Work out the finished part from the listing and answer in its coordinate system (mm). A direction names the side the tool comes from. Give positions to 0.01 mm unless a question says otherwise; leave off trailing zeros. Loops run counter-clockwise (first coordinate to the right, second up) from the corner with the lowest first, then second, coordinate; pieces in that order, holes last. Notation, with made-up numbers: (22, 29.5) - (52, 29.5) arc R6 cw to (52, 33.5) - close; hole circle Ø9 at (48, -1). An arc over 180 degrees is marked (long way). One line per item, written item: value.
from build123d import *

# Parameters (mm, degrees)
SKETCH_R  = 1.8288
PAD_DEPTH = 3


with BuildPart() as part:
    # Sketch → Pad (new body)
    with BuildSketch(Plane.XY):
        with BuildLine():
            Line((0, 100.6), (0, 1))
            ThreePointArc((0, 1), (0.292893, 0.292893), (1, 0))
            Line((1, 0), (14.748, 0))
            ThreePointArc((14.748, 0), (15.455107, 0.292893), (15.748, 1))
            Line((15.748, 12.7), (15.748, 1))
            ThreePointArc((22.352, 12.7), (19.05, 16.002), (15.748, 12.7))
            Line((22.352, 12.7), (22.352, 1))
            ThreePointArc((22.352, 1), (22.644893, 0.292893), (23.352, 0))
            Line((23.352, 0), (74.748, 0))
            ThreePointArc((74.748, 0), (75.455107, 0.292893), (75.748, 1))
            Line((75.748, 12.7), (75.748, 1))
            ThreePointArc((82.352, 12.7), (79.05, 16.002), (75.748, 12.7))
            Line((82.352, 12.7), (82.352, 1))
            ThreePointArc((82.352, 1), (82.644893, 0.292893), (83.352, 0))
            Line((83.352, 0), (97.1, 0))
            ThreePointArc((97.1, 0), (97.807107, 0.292893), (98.1, 1))
            Line((98.1, 1), (98.1, 24.9))
            ThreePointArc((99.1, 25.9), (98.392893, 25.607107), (98.1, 24.9))
            Line((99.1, 25.9), (119.2001, 25.9))
            ThreePointArc((119.2001, 25.9), (119.907207, 26.192893), (120.2001, 26.9))
            Line((120.2001, 26.9), (120.2001, 100.6))
            ThreePointArc((120.2001, 100.6), (119.907207, 101.307107), (119.2001, 101.6))
            Line((119.2001, 101.6), (1, 101.6))
            ThreePointArc((1, 101.6), (0.292893, 101.307107), (0, 100.6))
        make_face()
        with Locations((10.46, 95.25)):
            Circle(SKETCH_R, mode=Mode.SUBTRACT)
    extrude(amount=PAD_DEPTH)


solid = part.part
1. Section C-C (x = 79.05) is taken. Write down the section's boundary in (y, z).
Output:
outline: (16, 0) - (101.6, 0) - (101.6, 3) - (16, 3) - close
2. The mould has two halves that part along Y. Classify faces 4 (the cylindrical face through (12.15, 94.55, 1.48)), 5 (the flat face through (59, 52, 0)), 6 (the flat face through (49, 0, 1)): released by +Y, released by -Y, zero draft, split by the parting line, or undercut.
Output:
face 4: undercut
face 5: zero draft
face 6: released by -Y
3. Section A-A (x = 10.46) is taken. Write down the section's boundary in (y, z), and give its area (3 significant figures).
Output:
outline: (0, 0) - (93.42, 0) - (93.42, 3) - (0, 3) - close; (97.08, 0) - (101.6, 0) - (101.6, 3) - (97.08, 3) - close
area: 294 mm²
4. Flat-ended cylindrical pins translate along their axes: pin 1 Ø3.5 at (x, y) = (10.46, 95.25) entering from +Z; pin 2 Ø1.5 at (y, z) = (5.5, 1) entering from +X; pin 3 Ø4 at (x, y) = (98.5, 39) entering from -Z; pin 4 Ø1.5 at (x, z) = (108, 1.5) entering from -Y. Find the tip coordinate at first contact, or state that the pin passes through.
Output:
pin 1: passes through
pin 2: stops at x = 98.1
pin 3: stops at z = 0
pin 4: stops at y = 25.9
5. Section B-B (z = 1.85) is taken. Write down the section's boundary in (x, y).
Output:
outline: (0, 1) arc R1 ccw to (1, 0) - (14.75, 0) arc R1 ccw to (15.75, 1) - (15.75, 12.7) arc R3.3 cw to (22.35, 12.7) - (22.35, 1) arc R1 ccw to (23.35, 0) - (74.75, 0) arc R1 ccw to (75.75, 1) - (75.75, 12.7) arc R3.3 cw to (82.35, 12.7) - (82.35, 1) arc R1 ccw to (83.35, 0) - (97.1, 0) arc R1 ccw to (98.1, 1) - (98.1, 24.9) arc R1 cw to (99.1, 25.9) - (119.2, 25.9) arc R1 ccw to (120.2, 26.9) - (120.2, 100.6) arc R1 ccw to (119.2, 101.6) - (1, 101.6) arc R1 ccw to (0, 100.6) - close; hole circle Ø3.66 at (10.46, 95.25)
6. Find the intervals of material crossed by line 1 along X through (y, z) = (6, 0.2); line 2 along X through (y, z) = (95.25, 1.05); line 3 along Y through (x, z) = (10.46, 1.7), in increasing order.
Output:
line 1: x = 0 to 15.75, 22.35 to 75.75, 82.35 to 98.1
line 2: x = 0 to 8.63, 12.29 to 120.2
line 3: y = 0 to 93.42, 97.08 to 101.6
7. For faces 1 (the flat face through (61, 101.6, 1)), 2 (the flat face through (98.1, 13, 1)), 3 (the flat face through (82.352, 7, 1)), determine the directions among +Z, -Z, +X, -X, +Y, -Y from which every point of the face is accessible in a straight line to the end or side of a thin tool.
Output:
face 1: +Z, -Z, +X, -X, +Y
face 2: +Z, -Z, +X, -Y
face 3: +Z, -Z, -Y
